Check sheet for the drawn part. Datum: minimum x, y, z corner. Units: mm. A direction names the side the tool comes from. Round coordinates to 2 decimals unless told otherwise and drop trailing zeros. Write each loop counter-clockwise with the first axis right and the second up, starting at its lowest first coordinate (ties: lowest second). Pieces come first, ordered by that corner, then holes.
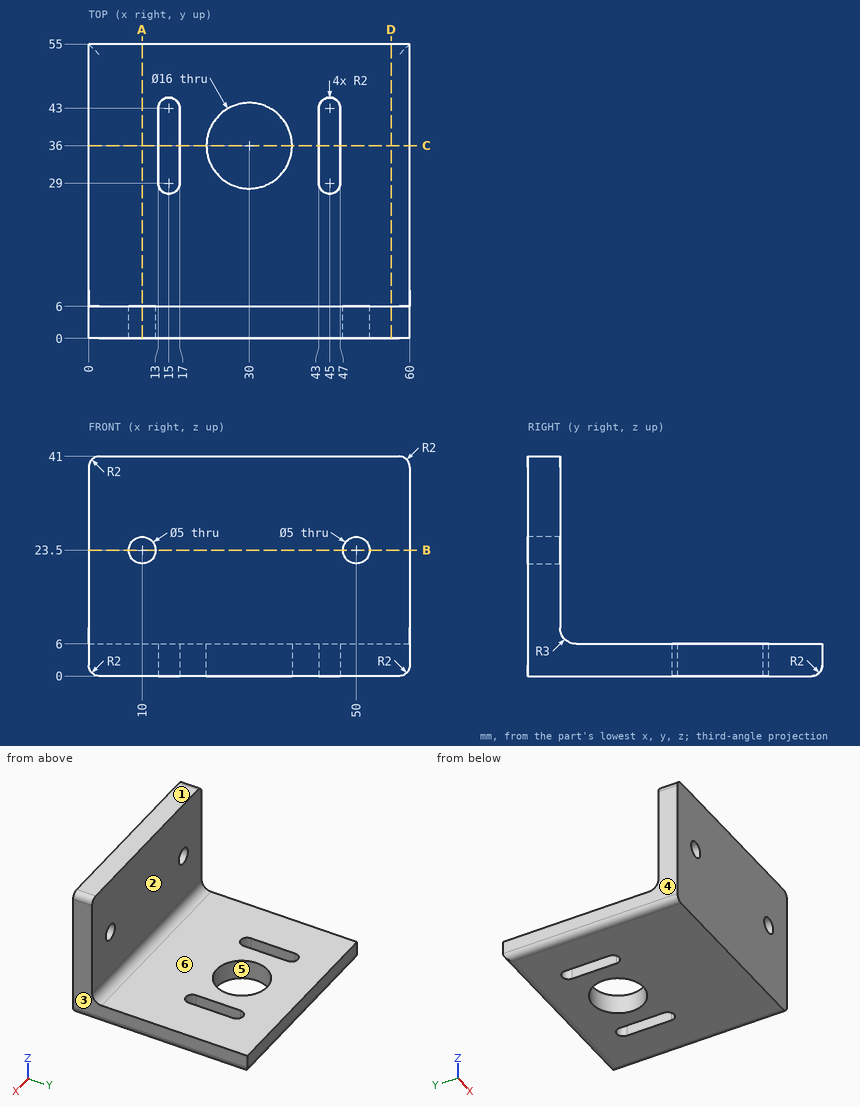
Q1. Tool access check on the marked faces 1 and 2. Record the directions out of +Z, -Z, +X, -X, +Y, -Y that give a thin tool (end or side, any length) a straight path to the whole face; none if there is none.
Recorded:
face 1: +Z, +X, -X, +Y, -Y
face 2: +Z, +X, -X, +Y
Q2. Sectioned sample at B-B (z = 23.5). Enter the section's corners in (x, y), plus the area to 3 significant figures.
Recorded:
outline: (0, 0) - (7.5, 0) - (7.5, 6) - (0, 6) - close; (12.5, 0) - (47.5, 0) - (47.5, 6) - (12.5, 6) - close; (52.5, 0) - (60, 0) - (60, 6) - (52.5, 6) - close
area: 300 mm2
Q3. Depth check by flat-ended pin: P1, Ø5, axis at y = 34, z = 4, coming from the -X side; P2, Ø1, axis at x = 44, y = 8, coming from the +Z side; P3, Ø14, axis at x = 36.5, y = 30, coming from the +Z side; P4, Ø8, axis at x = 10, z = 23.5, coming from the +Y side. Enter the tip coordinate at first touch or a pass-through.
Recorded:
P1: stops at x = 0
P2: stops at z = 6.4
P3: stops at z = 6
P4: stops at y = 6
Q4. Release check for a two-part mould opening along X. For the marked faces 3, 4, 5 and 6 record: released by +X, released by -X, zero draft, split by the parting line, or undercut.
Recorded:
face 3: released by +X
face 4: released by -X
face 5: undercut
face 6: zero draft
Q5. Sectioned sample at D-D (x = 56.5). Enter the section's corners in (y, z), plus the area to 3 significant figures.
Recorded:
outline: (0, 0) - (53, 0) arc R2 ccw to (55, 2) - (55, 6) - (9, 6) arc R3 cw to (6, 9) - (6, 41) - (0, 41) - close
area: 541 mm2
Q6. Sectioned sample at A-A (x = 10). Enter the section's corners in (y, z).
Recorded:
outline: (0, 0) - (53, 0) arc R2 ccw to (55, 2) - (55, 6) - (9, 6) arc R3 cw to (6, 9) - (6, 21) - (0, 21) - close; (0, 26) - (6, 26) - (6, 41) - (0, 41) - close
Q7. Sectioned sample at C-C (y = 36). Enter the section's corners in (x, z).
Recorded:
outline: (0, 2) arc R2 ccw to (2, 0) - (13, 0) - (13, 6) - (0, 6) - close; (17, 0) - (22, 0) - (22, 6) - (17, 6) - close; (38, 0) - (43, 0) - (43, 6) - (38, 6) - close; (47, 0) - (58, 0) arc R2 ccw to (60, 2) - (60, 6) - (47, 6) - close
Q8. Material ranges on line 1 along X through (y, z) = (4.6, 23.5); line 2 along Y through (x, z) = (30, 4); line 3 along X through (y, z) = (1, 23), recorded low to high.
Recorded:
line 1: x = 0 to 7.5, 12.5 to 47.5, 52.5 to 60
line 2: y = 0 to 28, 44 to 55
line 3: x = 0 to 7.55, 12.45 to 47.55, 52.45 to 60
